Build history of the part. All positions in model axes, mm. Face numbers are marked on the shaded views. Coordinates: 2 decimals unless noted, no trailing zeros. Order: outer loops, then holes, each group sorted by start corner. A loop starts at its lowest first (then second) coordinate and runs counter-clockwise, first axis right, second up. Notation, with made-up numbers: (72.5, -32) - (89.5, -32) arc R22 ccw to (89.5, -12) - close; hole circle Ø9 at (3, 57). An arc over 180 degrees is marked (long way). Write each question's results on one line, items separated by ' | '. Start each with the question number.
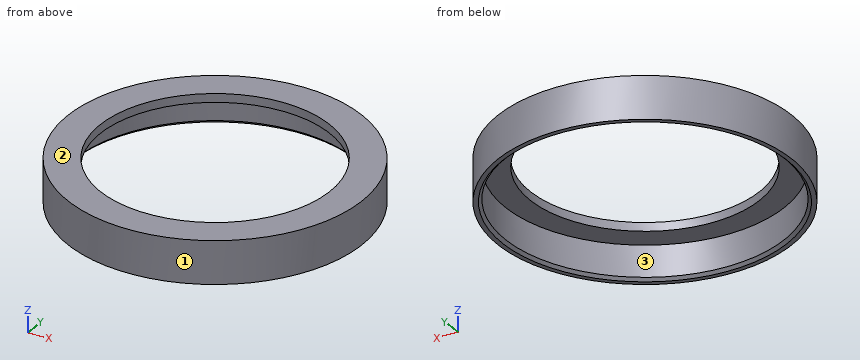
from build123d import *

# Parameters (mm, degrees)
F0_R     = 64.77
F0_R_2   = 51
F1_DEPTH = 3.81
F2_R     = 65.3415
F2_R_2   = 61.976
F3_DEPTH = 19
F4_SIZE  = 1.27


with BuildPart() as f1:
    # F0 (on Top) → F1 (new body)
    with BuildSketch(Plane.XY):
        Circle(F0_R)
        Circle(F0_R_2, mode=Mode.SUBTRACT)
    extrude(amount=-F1_DEPTH)

    # F2 (on face) → F3 (join)
    with BuildSketch(Plane.XY):
        Circle(F2_R)
        Circle(F2_R_2, mode=Mode.SUBTRACT)
    extrude(amount=-F3_DEPTH)

    # F4
    f4_edges = [f1.edges().sort_by_distance(p)[0] for p in [
        (-61.976, 0, -19),
    ]]
    chamfer(f4_edges, length=F4_SIZE)


solid = f1.part
Item 1: Flat gauge pins, fed straight in: P1, Ø6, axis at y = -32, z = -13, coming from the +X side; P2, Ø8, axis at x = -29.5, z = -3.5, coming from the -Y side; P3, Ø8, axis at y = 20, z = -11.5, coming from the +X side. Where does each tip first touch, or does it go through?
Item 2: Slice it at D-D (z = -2.25). Write the cut outline in (x, y).
Item 3: Slice it at C-C (z = -15). Write the cut outline in (x, y), then the cut area to 3 significant figures.
Item 4: Probe probe 1 along Y at (x, z) = (0, -1.6); probe 2 along Y at (x, z) = (0, -8.75); probe 3 along Z at (x, y) = (-29, 49.5). List the from-to ranges inside material, lowest first.
Item 5: Pull direction X, two halves, no side cores. Call the marked faces 1, 2 and 3: released by +X, released by -X, zero draft, split by the parting line, or undercut.
Item 6: Slice it at A-A (y = 0). Write the cut outline in (x, z), then the cut area to 3 significant figures.
Resolved:
1) P1: x = 58.55 | P2: y = -60.16 | P3: x = 63.35
2) outline: circle Ø130.68 at (0, 0); hole circle Ø102 at (0, 0)
3) outline: circle Ø130.68 at (0, 0); hole circle Ø123.95 at (0, 0) | area: 1,350 mm^2
4) probe 1: -65.34 to -51, 51 to 65.34 | probe 2: -65.34 to -61.98, 61.98 to 65.34 | probe 3: -3.81 to 0
5) face 1: split by the parting line | face 2: zero draft | face 3: undercut
6) outline: (-65.34, -19) - (-63.25, -19) - (-61.98, -17.73) - (-61.98, -3.81) - (-51, -3.81) - (-51, 0) - (-65.34, 0) - close; (51, -3.81) - (61.98, -3.81) - (61.98, -17.73) - (63.25, -19) - (65.34, -19) - (65.34, 0) - (51, 0) - close | area: 210 mm^2
